from build123d import *

# Parameters (mm, degrees)
SKETCH1_R           = 3.2639
SKETCH1_R_2         = 7.9375
SKETCH1_R_3         = 4.191
BOSS_EXTRUDE4_DEPTH = 3.175


with BuildPart() as part:
    # Sketch1 → Boss-Extrude4 (new body)
    with BuildSketch(Plane(origin=(0, 0, 0), x_dir=(1, 0, 0), z_dir=(0, 1, 0))):
        with BuildLine():
            Line((27.261215437, -20.782448937), (109.864793621, -8.887225298))
            ThreePointArc((109.864793621, -8.887225298), (113.829824864, -7.2878294), (116.60566957, -4.036025875))
            Line((116.60566957, -4.036025875), (133.726592386, 29.98785526))
            ThreePointArc((133.726592386, 29.98785526), (132.627611185, 40.61059676), (122.521356715, 44.06226552))
            Line((122.521356715, 44.06226552), (-3.247611444, 13.260609947))
            ThreePointArc((-3.247611444, 13.260609947), (-13.651443786, 0.16981992), (-3.576471569, -13.175720374))
            Line((-3.576471569, -13.175720374), (23.629267956, -20.560557875))
            ThreePointArc((23.629267956, -20.560557875), (25.433883661, -20.857413504), (27.261215437, -20.782448937))
        make_face()
        with Locations(Location((25.981421816, -11.895223639, 0), (0, 0, 270))):
            Circle(SKETCH1_R, mode=Mode.SUBTRACT)
        with Locations(Location((0, 0, 0), (0, 0, 270))):
            Circle(SKETCH1_R_2, mode=Mode.SUBTRACT)
        with BuildLine():
            ThreePointArc((100.723144875, 4.337266328), (99.62721378, 0.615395192), (100.203869733, -3.221381793))
            Line((100.203869733, -3.221381793), (34.930946987, -12.620926349))
            ThreePointArc((34.930946987, -12.620926349), (26.528959971, -2.933033774), (17.010113752, -11.526066709))
            Line((17.010113752, -11.526066709), (9.750952301, -9.555610157))
            ThreePointArc((9.750952301, -9.555610157), (13.651443786, -0.16981992), (9.985636063, 9.310092839))
            Line((9.985636063, 9.310092839), (79.071831614, 26.229760952))
            Line((79.071831614, 26.229760952), (100.723144875, 4.337266328))
        make_face(mode=Mode.SUBTRACT)
        with Locations(Location((108.585, 0, 0), (0, 0, 270))):
            Circle(SKETCH1_R, mode=Mode.SUBTRACT)
        with BuildLine():
            Line((104.335087932, 7.90941797), (84.823475635, 27.638376771))
            Line((84.823475635, 27.638376771), (114.98908268, 35.026134276))
            ThreePointArc((114.98908268, 35.026134276), (117.570132445, 27.752761279), (124.58688197, 24.538885311))
            Line((124.58688197, 24.538885311), (115.260501822, 6.004858086))
            ThreePointArc((115.260501822, 6.004858086), (110.126982004, 8.845503757), (104.335087932, 7.90941797))
        make_face(mode=Mode.SUBTRACT)
        with Locations(Location((124.877763158, 34.440613651, 0), (0, 0, 270))):
            Circle(SKETCH1_R_3, mode=Mode.SUBTRACT)
    extrude(amount=-BOSS_EXTRUDE4_DEPTH)


solid = part.part
Input: part model. Units: mm. Frame: model coordinates. A direction names the side the tool comes from. Coordinates: 2 decimals unless noted, no trailing zeros. Loops run counter-clockwise (first coordinate to the right, second up) from the corner with the lowest first, then second, coordinate; pieces in that order, holes last. Notation, with made-up numbers: (0.25, 85) -> (25.25, 85) arc R14 ccw to (25.25, 107) -> close; hole circle Ø4 at (64, -34.5). An arc over 180 degrees is marked (long way). One line per item, written item: value.
(1) Ray query, line 1 along Z through (x, y) = (90.5, -1.4); line 2 along X through (y, z) = (-1.4, 0); line 3 along Z through (x, y) = (88.5, -0.2). Return the intervals inside material, ascending.
Answer below:
line 1: z = -36.22 to -29.03, -21.9 to -14.67, 4.62 to 11.68
line 2: x = -13.65 to -7.94, 7.94 to 13.65, 99.61 to 105.32, 111.85 to 118.64
line 3: z = -35.73 to -28.54, -23.92 to -16.7, 4.91 to 11.96
(2) Draft query along X for faces 3 (the face through (113.781, -1.565, 7.323)), 4 (the face through (117.496, -1.565, -27.835)), 5 (the face through (60.517, -1.565, -28.877)). Return one class per face: pulls with the +X half, pulls with the -X half, needs draft (parallel to the pull), parting line crosses it, or undercut.
Answer below:
face 3: pulls with the +X half
face 4: undercut
face 5: pulls with the -X half
(3) Set-up query: faces 1 (the face through (-13.646, -1.565, -0.422)), 2 (the face through (94.716, -1.565, -17.636)). Return all of +Z, -Z, +X, -X, +Y, -Y with unobstructed straight access to the full face (end or side cutting, diameter ignored); none if empty.
Answer below:
face 1: -X, +Y, -Y
face 2: +Y, -Y
(4) Pin query (flat end, axial travel): pin 1 Ø1.5 at (x, z) = (7.5, 3.5) entering from +Y; pin 2 Ø1.5 at (y, z) = (-1.5, -11) entering from -X; pin 3 Ø1 at (y, z) = (-1, 5) entering from -X; pin 4 Ø1 at (y, z) = (-2.5, -18) entering from +X. Return the tip coordinate at first contact, or that it passes through.
Answer below:
pin 1: stops at y = 0
pin 2: stops at x = -9.02
pin 3: stops at x = -12.89
pin 4: stops at x = 127.95
(5) Cut plane D-D (x = 70). Output: boundary loops of the cut face in (y, z) (3 decimals).
Answer below:
outline: (-3.175, -31.199) -> (0, -31.199) -> (0, -24.008) -> (-3.175, -24.008) -> close; (-3.175, 7.571) -> (0, 7.571) -> (0, 14.628) -> (-3.175, 14.628) -> close
(6) Cut plane B-B (z = 0). Output: boundary loops of the cut face in (x, y) (1 decimal).
Answer below:
outline: (-13.7, -3.2) -> (-7.9, -3.2) -> (-7.9, 0) -> (-13.7, 0) -> close; (7.9, -3.2) -> (13.7, -3.2) -> (13.7, 0) -> (7.9, 0) -> close; (99.6, -3.2) -> (105.3, -3.2) -> (105.3, 0) -> (99.6, 0) -> close; (111.8, -3.2) -> (118.6, -3.2) -> (118.6, 0) -> (111.8, 0) -> close
(7) Cut plane C-C (y = -1.45). Output: boundary loops of the cut face in (x, z) (1 decimal), then the cut area to 3 significant figures.
Answer below:
outline: (-3.6, 13.2) arc R13.7 ccw to (-3.2, -13.3) -> (122.5, -44.1) arc R9.9 ccw to (133.7, -30) -> (116.6, 4) arc R9 ccw to (109.9, 8.9) -> (27.3, 20.8) arc R9 ccw to (23.6, 20.6) -> close; hole circle Ø15.9 at (0, 0); hole (9.8, 9.6) arc R13.7 cw to (10, -9.3) -> (79.1, -26.2) -> (100.7, -4.3) arc R9 cw to (100.2, 3.2) -> (34.9, 12.6) arc R9 cw (long way) to (17, 11.5) -> close; hole circle Ø6.5 at (26, 11.9); hole (84.8, -27.6) -> (115, -35) arc R9.9 cw to (124.6, -24.5) -> (115.3, -6) arc R9 cw to (104.3, -7.9) -> close; hole circle Ø6.5 at (108.6, 0); hole circle Ø8.4 at (124.9, -34.4)
area: 2,750 mm2
(8) Cut plane A-A (x = 0). Output: boundary loops of the cut face in (y, z) (1 decimal).
Answer below:
outline: (-3.2, -14.1) -> (0, -14.1) -> (0, -7.9) -> (-3.2, -7.9) -> close; (-3.2, 7.9) -> (0, 7.9) -> (0, 14.1) -> (-3.2, 14.1) -> close
